```python
from build123d import *

# Parameters (mm, degrees)
F0_W           = 150
F0_H           = 30
F1_DEPTH       = 1125
F3_D           = 5.5
F3_CBORE_D     = 9.75
F3_CBORE_DEPTH = 5
F4_W           = 45
F4_H           = 15
F5_DEPTH       = 1125.001
F7_D           = 6.6
F7_DEPTH       = 9
F7_TIP         = 1.9828400428


with BuildPart() as f1:
    # F0 (on Front) → F1 (new body)
    with BuildSketch(Plane.XZ):
        Rectangle(F0_W, F0_H)
    extrude(amount=F1_DEPTH)

    # F3 (through all)
    with Locations(Plane.XY.offset(15)):
        with Locations((-67, -1092), (-67, -1038), (-43, -1038), (-43, -1092), (43, -1092), (67, -1092), (67, -1038), (43, -1038), (-67, -577), (-43, -577), (-43, -523), (-67, -523), (43, -523), (67, -523), (67, -577), (43, -577), (43, -62), (43, -8), (67, -8), (67, -62), (-43, -62), (-67, -62), (-67, -8), (-43, -8)):
            CounterBoreHole(F3_D / 2, F3_CBORE_D / 2, F3_CBORE_DEPTH)

    # F4 (on face) → F5 (cut, through all)
    with BuildSketch(Plane.XZ.offset(1125)):
        with Locations((-52.5, -7.5)):
            Rectangle(F4_W, F4_H)
        with Locations((52.5, -7.5)):
            Rectangle(F4_W, F4_H)
    extrude(amount=-F5_DEPTH, mode=Mode.SUBTRACT)

    # F7
    with Locations(Plane.YZ.offset(75)):
        with Locations((-1025, 7.5), (-825, 7.5), (-625, 7.5), (-425, 7.5), (-225, 7.5)):
            Hole(F7_D / 2, depth=F7_DEPTH)
            with Locations((0, 0, -(F7_DEPTH + F7_TIP / 2))):  # 118° drill point
                Cone(0, F7_D / 2, F7_TIP, mode=Mode.SUBTRACT)


solid = f1.part
```
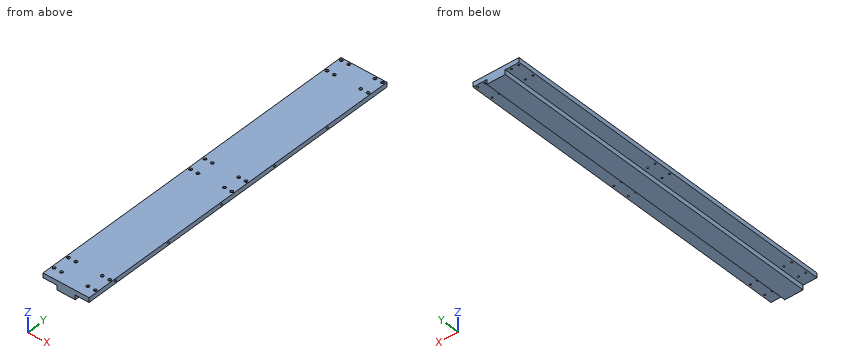
Part model, mm, in its own coordinate system. Round coordinates to 2 decimals unless told otherwise and drop trailing zeros. Write each loop counter-clockwise with the first axis right and the second up, starting at its lowest first coordinate (ties: lowest second). Pieces come first, ordered by that corner, then holes. Notation, with made-up numbers: M 29,55.5 L 70,55.5 A10 ccw 70,67.5 Z; hole C 26.5,-24 d7. An arc over 180 degrees is marked long. One line per question, with ' | ' between items.
(1) Pin check, flat tips, straight feed: pin 1 (6 mm diameter, centred on y = -152, z = -4, fed in from -X); pin 2 (3 mm diameter, centred on x = 49.5, y = -511, fed in from -Z); pin 3 (3 mm diameter, centred on x = -42, y = -62.5, fed in from +Z); pin 4 (8 mm diameter, centred on x = 42.5, y = -1092.5, fed in from +Z). Stop position of each tip, or through.
Answer key:
pin 1: stops at x = -30 | pin 2: stops at z = 0 | pin 3: passes through | pin 4: stops at z = 10
(2) Saw through at A-A on y = -544. Write the cut outline in (x, z), then the cut area to 3 significant figures.
Answer key:
outline: M -75,0 L -30,0 L -30,-15 L 30,-15 L 30,0 L 75,0 L 75,15 L -75,15 Z | area: 3,150 mm^2
(3) Probe line 1 along Y through (x, z) = (71.75, 7.5); line 2 along X through (y, z) = (-577, 8.25); line 3 along Z through (x, y) = (-55.5, -397.5). List the from-to ranges inside material, lowest first.
Answer key:
line 1: y = -1125 to -1028.3, -1021.7 to -828.3, -821.7 to -628.3, -621.7 to -428.3, -421.7 to -228.3, -221.7 to 0 | line 2: x = -75 to -69.75, -64.25 to -45.75, -40.25 to 40.25, 45.75 to 64.25, 69.75 to 75 | line 3: z = 0 to 15
